Check sheet for the modelled part. Datum: model origin and axes. Units: mm. A direction names the side the tool comes from. Give positions to 0.01 mm unless a question says otherwise; leave off trailing zeros. Write each loop counter-clockwise with the first axis right and the second up, starting at its lowest first coordinate (ties: lowest second). Pieces come first, ordered by that corner, then holes. Notation, with made-up numbers: M 47.25,71 L 93.25,71 A21 ccw 93.25,94 Z; hole C 45,50.25 d3. An arc over 180 degrees is marked long. Use CSV: the item, a comma, the result in double quotes. Start each with the question number.
1. Cross-section at A-A, the plane x = 0. Enter the section's corners in (y, z).
2. Mould release check, pull along X, two halves, no side actions. Record for faces 1 (the face through (-1.216, 1.115, 0.479)), 2 (the face through (0, -4, 5)), 3 (the face through (-5, -4, 3)): +X half, -X half, draft (parallel to the pull), parting line (faces both ways), or undercut.
3. Cross-section at C-C, the plane x = 3.75. Enter the section's corners in (y, z), and give its area (3 significant figures).
4. Scan lines: line 1 (X direction, y = 0, z = 3.65); line 2 (X direction, y = 0, z = 0.9); line 3 (Y direction, x = -2, z = 10.75). Record each from-to range of solid material in increasing order.
5. Cross-section at B-B, the plane z = 10. Enter the section's corners in (x, y), and give its area (3 significant figures).
6. Cross-section at D-D, the plane z = 1.75. Enter the section's corners in (x, y).
7. Depth check by flat-ended pin: P1, Ø4, axis at x = 0, y = 0, coming from the +Z side; P2, Ø6, axis at y = -0.5, z = 6, coming from the +X side; P3, Ø3, axis at x = -1.5, y = 1.5, coming from the +Z side; P4, Ø3, axis at x = 0, z = 10, coming from the +Y side. Enter the tip coordinate at first touch or a pass-through.
8. Access from +Z, -Z, +X, -X, +Y, -Y to the whole of each face (thin tool, end or side, straight path). Record for faces 4 (the face through (-1, -5.5, 8)), 5 (the face through (0, -7, 0)), 6 (the face through (-0.1, 3.9, -0.5)), 7 (the face through (1, -2, 2)).
from build123d import *

# Parameters (mm, degrees)
CYLINDER006_R      = 1.65
CYLINDER006_DEPTH  = 10
CYLINDER007_R      = 3.5
CYLINDER007_DEPTH  = 10
CYLINDER008_R      = 1.9
CYLINDER008_DEPTH  = 10
BOX016_W           = 10
BOX016_H           = 16.5
BOX016_DEPTH       = 5
BOX017_W           = 10
BOX017_H           = 7.8
BOX017_DEPTH       = 2
CHAMFER003015_SIZE = 1
BOX015_W           = 10
BOX015_H           = 4.5
BOX015_DEPTH       = 15
CHAMFER003016_SIZE = 0.4
CHAMFER003017_SIZE = 2


with BuildPart() as cylinder006:
    # Cylinder006 → Cylinder006 (new body)
    with BuildSketch(Plane.XY.offset(-4)):
        Circle(CYLINDER006_R)
    extrude(amount=CYLINDER006_DEPTH)


with BuildPart() as fusion011:
    # Cylinder007 → Cylinder007 (new body)
    with BuildSketch(Plane.XY.offset(2)):
        Circle(CYLINDER007_R)
    extrude(amount=CYLINDER007_DEPTH)

    # Fusion011: union Cylinder006
    add(cylinder006.part)


with BuildPart() as cylinder008:
    # Cylinder008 → Cylinder008 (new body)
    with BuildSketch(Plane(origin=(0, -12, 10), x_dir=(1, 0, 0), z_dir=(0, 1, 0))):
        Circle(CYLINDER008_R)
    extrude(amount=CYLINDER008_DEPTH)


with BuildPart() as cube016:
    # Box016 → Box016 (new body)
    with BuildSketch(Plane(origin=(-5, -9.5, 0), x_dir=(1, 0, 0), z_dir=(0, 0, 1))):
        with Locations((5, 8.25)):
            Rectangle(BOX016_W, BOX016_H)
    extrude(amount=BOX016_DEPTH)


with BuildPart() as chamfer003015:
    # Box017 → Box017 (new body)
    with BuildSketch(Plane(origin=(-5, -3.9, -1), x_dir=(1, 0, 0), z_dir=(0, 0, 1))):
        with Locations((5, 3.9)):
            Rectangle(BOX017_W, BOX017_H)
    extrude(amount=BOX017_DEPTH)

    # Chamfer003015
    chamfer003015_edges = [chamfer003015.edges().sort_by_distance(p)[0] for p in [
        (0, -3.9, -1),
    ]]
    chamfer(chamfer003015_edges, length=CHAMFER003015_SIZE)


with BuildPart() as back_panel_support:
    # Box015 → Box015 (new body)
    with BuildSketch(Plane(origin=(-5, -10, 0), x_dir=(1, 0, 0), z_dir=(0, 0, 1))):
        with Locations((5, 2.25)):
            Rectangle(BOX015_W, BOX015_H)
    extrude(amount=BOX015_DEPTH)

    # Fusion012: union Cube016, Chamfer003015
    add(cube016.part)
    add(chamfer003015.part)

    # Chamfer003016
    chamfer003016_edges = [back_panel_support.edges().sort_by_distance(p)[0] for p in [
        (0, -10, 15),
        (0, -10, 0),
        (0, 7, 0),
    ]]
    chamfer(chamfer003016_edges, length=CHAMFER003016_SIZE)

    # Chamfer003017
    chamfer003017_edges = [back_panel_support.edges().sort_by_distance(p)[0] for p in [
        (0, -5.5, 15),
        (0, 7, 5),
    ]]
    chamfer(chamfer003017_edges, length=CHAMFER003017_SIZE)

    # Cut008004003004014002002005003004002: cut Cylinder008
    add(cylinder008.part, mode=Mode.SUBTRACT)

    # Cut008004003004014002002005003004003: cut Fusion011
    add(fusion011.part, mode=Mode.SUBTRACT)


solid = back_panel_support.part
Worked answers:
1,outline,"M -10,0.4 L -9.6,0 L -3.9,0 L -2.9,-1 L -1.65,-1 L -1.65,2 L -3.5,2 L -3.5,5 L -5.5,5 L -5.5,8.1 L -10,8.1 Z; M -10,11.9 L -5.5,11.9 L -5.5,13 L -7.5,15 L -9.6,15 L -10,14.6 Z; M 1.65,-1 L 3.9,-1 L 3.9,0 L 6.6,0 L 7,0.4 L 7,3 L 5,5 L 3.5,5 L 3.5,2 L 1.65,2 Z"
2,face 1,"undercut"
2,face 2,"draft"
2,face 3,"-X half"
3,outline,"M -10,0.4 L -9.6,0 L -3.9,0 L -2.9,-1 L 3.9,-1 L 3.9,0 L 6.6,0 L 7,0.4 L 7,3 L 5,5 L -5.5,5 L -5.5,13 L -7.5,15 L -9.6,15 L -10,14.6 Z"
3,area,"133 mm^2"
4,line 1,"x = -5 to -3.5, 3.5 to 5"
4,line 2,"x = -5 to -1.65, 1.65 to 5"
4,line 3,"y = -10 to -5.5"
5,outline,"M -5,-10 L -1.9,-10 L -1.9,-5.5 L -5,-5.5 Z; M 1.9,-10 L 5,-10 L 5,-5.5 L 1.9,-5.5 Z"
5,area,"27.9 mm^2"
6,outline,"M -5,-10 L 5,-10 L 5,7 L -5,7 Z; hole C 0,0 d3.3"
7,P1,"stops at z = 2"
7,P2,"stops at x = 5"
7,P3,"stops at z = 5"
7,P4,"passes through"
8,face 4,"+Z, +X, -X, +Y"
8,face 5,"-Z, +X, -X, -Y"
8,face 6,"-Z, +X, -X, +Y"
8,face 7,"+Z"
